Here's the drawing with two shaded views (mm, measured from the low corner). I have some questions. Give positions to 0.01 mm unless a question says otherwise; leave off trailing zeros. Write each loop counter-clockwise with the first axis right and the second up, starting at its lowest first coordinate (ties: lowest second). Pieces come first, ordered by that corner, then holes.
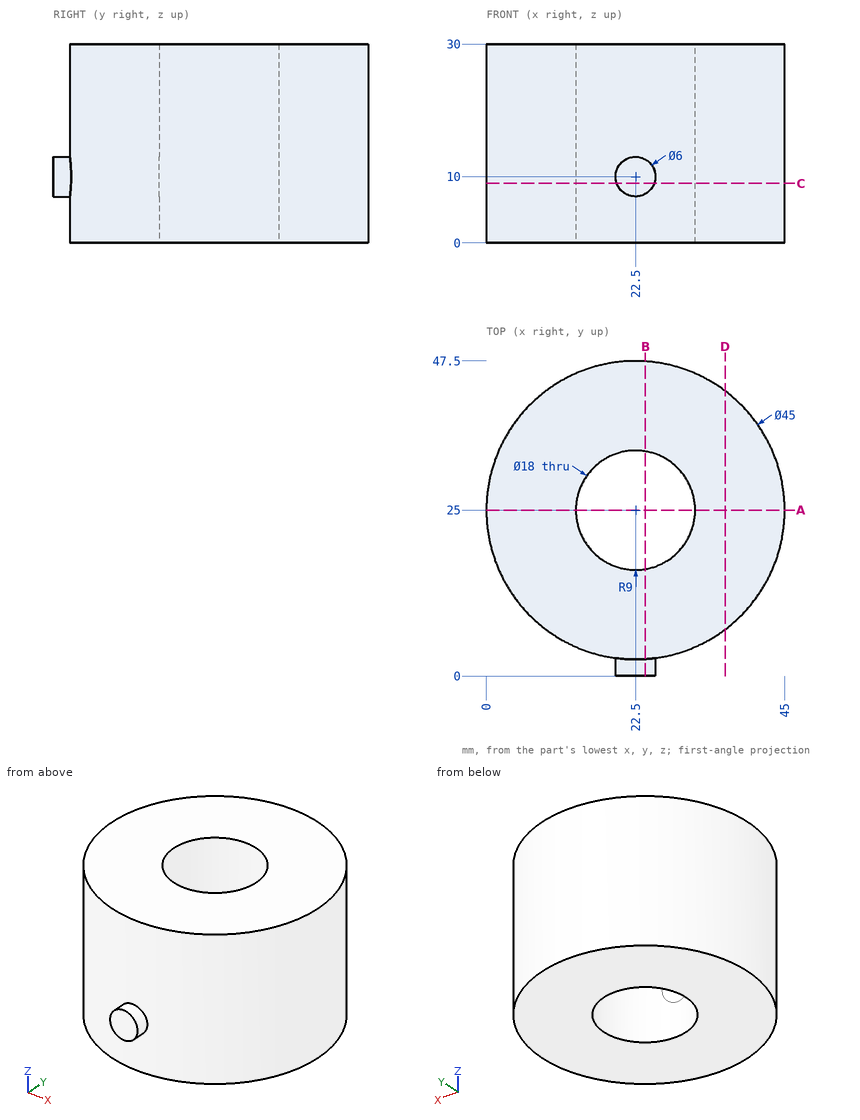
(1) If I drill on L1, parallel to Y at x = 22, z = 9; L2, parallel to Y at x = 22, z = 23.5; L3, parallel to X at y = 22.5, z = 8.5, over which ranges is the centre line in solid material (lowest first)?
Returned:
L1: y = 0 to 16.01, 33.99 to 47.49
L2: y = 2.51 to 16.01, 33.99 to 47.49
L3: x = 0.14 to 13.85, 31.15 to 44.86
(2) Imagine slicing it at A-A, the plane y = 25. Write out the boundary of the cut face in (x, z), plus the area to 3 significant figures.
Returned:
outline: (0, 0) - (13.5, 0) - (13.5, 30) - (0, 30) - close; (31.5, 0) - (45, 0) - (45, 30) - (31.5, 30) - close
area: 810 mm2
(3) Imagine slicing it at B-B, the plane x = 24. Write out the boundary of the cut face in (y, z).
Returned:
outline: (0, 7.4) - (2.55, 7.4) - (2.55, 0) - (16.13, 0) - (16.13, 30) - (2.55, 30) - (2.55, 12.6) - (0, 12.6) - close; (33.87, 0) - (47.45, 0) - (47.45, 30) - (33.87, 30) - close
(4) Imagine slicing it at C-C, the plane z = 9. Write out the boundary of the cut face in (x, y), plus the area to 3 significant figures.
Returned:
outline: (19.67, 0) - (25.33, 0) - (25.33, 2.68) arc R22.5 ccw (long way) to (19.67, 2.68) - close; hole circle Ø18 at (22.5, 25)
area: 1,350 mm2
(5) Will these pins go through, and if not, where does the flat tip stop? P1, Ø5, axis at y = 28.5, z = 15, coming from the +X side; P2, Ø11, axis at x = 22.5, y = 25, coming from the -Z side; P3, Ø1.5, axis at y = 32, z = 13.5, coming from the +X side; P4, Ø12, axis at x = 40.5, z = 21.5, coming from the +Y side.
Returned:
P1: stops at x = 44.98
P2: passes through
P3: stops at x = 44.11
P4: stops at y = 44.03
(6) Imagine slicing it at D-D, the plane x = 36. Write out the boundary of the cut face in (y, z).
Returned:
outline: (7, 0) - (43, 0) - (43, 30) - (7, 30) - close
